from build123d import *

# Parameters (mm, degrees)
F1_DEPTH = 25.4
F2_R     = 5.08
F3_R     = 5.08
F4_R     = 8.3693802945
F5_DEPTH = 99.314


with BuildPart() as f1:
    # F0 (on Front) → F1 (new body, symmetric)
    with BuildSketch(Plane.XZ):
        Polygon((37.378333509, -16.5805853903), (37.378333509, 16.5805853903), (9.2585918344, 16.5805853903), (-10.9242624321, 16.5805853903), (-37.378333509, 16.5805853903), (-37.378333509, -16.5805853903), align=None)
        with BuildLine():
            Line((-10.9242624321, 16.5805853903), (9.2585918344, 16.5805853903))
            ThreePointArc((9.2585918344, 16.5805853903), (16.1053006485, 34.9702005239), (33.311298198, 44.4046594203))
            Line((33.311298198, 44.4046594203), (33.311298198, 64.7116564196))
            ThreePointArc((33.311298198, 64.7116564196), (1.814383096, 49.2661510986), (-10.9242624321, 16.5805853903))
        make_face()
        with BuildLine():
            Line((33.311298198, 72.2287222743), (33.311298198, 64.7116564196))
            ThreePointArc((33.311298198, 64.7116564196), (57.7910346378, 60.35800431), (76.8620222807, 44.4046594203))
            Line((76.8620222807, 44.4046594203), (76.8620222807, 72.2287222743))
            Line((76.8620222807, 72.2287222743), (33.311298198, 72.2287222743))
        make_face()
        with BuildLine():
            Line((33.311298198, 64.7116564196), (33.311298198, 44.4046594203))
            Line((33.311298198, 44.4046594203), (76.8620222807, 44.4046594203))
            ThreePointArc((76.8620222807, 44.4046594203), (57.7910346378, 60.35800431), (33.311298198, 64.7116564196))
        make_face()
    extrude(amount=F1_DEPTH, both=True)

    # F2
    f2_edges = [f1.edges().sort_by_distance(p)[0] for p in [
        (-37.378334, -25.4, 0),
        (37.378334, -25.4, 0),
        (37.378334, 25.4, 0),
        (-37.378334, 25.4, 0),
    ]]
    fillet(f2_edges, radius=F2_R)

    # F3
    f3_edges = [f1.edges().sort_by_distance(p)[0] for p in [
        (9.258592, 0, 16.580585),
        (-10.924262, 0, 16.580585),
        (33.311298, 0, 72.228722),
        (76.862022, 0, 72.228722),
        (76.862022, 0, 44.404659),
    ]]
    fillet(f3_edges, radius=F3_R)

    # F4 (on face) → F5 (cut)
    with BuildSketch(Plane(origin=(0, 0, -16.5805853903), x_dir=(1, 0, 0), z_dir=(0, 0, -1))):
        Circle(F4_R)
    extrude(amount=-F5_DEPTH, mode=Mode.SUBTRACT)


solid = f1.part
Check sheet for the modelled part. Datum: model origin and axes. Units: mm. A direction names the side the tool comes from. Give positions to 0.01 mm unless a question says otherwise; leave off trailing zeros. Order: outer loops, then holes, each group sorted by start corner. A loop starts at its lowest first (then second) coordinate and runs counter-clockwise, first axis right, second up. Notation, with made-up numbers: M 76,40.25 L 82,40.25 A25 ccw 82,58.25 Z; hole C 5,-32 d4. An arc over 180 degrees is marked long. Answer as CSV lines item,"result". Start each with the question number.
Item 1: Thickness scan on line 1 (Y direction, x = 0, z = 25); line 2 (X direction, y = 0, z = 12); line 3 (X direction, y = 0, z = 22.5). Record the ranges inside material, lowest first. Write a range as [from, to].
Item 2: Cross-section at D-D on y = 17.5. Enter the section's corners in (x, z), plus the area to 3 significant figures.
Item 3: Mould release check, pull along Y, two halves, no side actions. Record for faces 5 (the face through (9, -25.4, 28)), 6 (the face through (33.311, 0, 66)), 7 (the face through (7.983, -2.514, 18.808)), 8 (the face through (-35.9, 23.9, -0.2)): +Y half, -Y half, draft (parallel to the pull), parting line (faces both ways), or undercut.
Item 4: Tool access check on faces 1 (the face through (-37.378, 0, 0)), 2 (the face through (26, 0, 16.581)), 3 (the face through (35.9, 23.9, 0.2)), 4 (the face through (37.378, 0, 0)). Record the directions out of +Z, -Z, +X, -X, +Y, -Y that give a thin tool (end or side, any length) a straight path to the whole face; none if there is none.
Item 5: Cross-section at C-C on x = 0. Enter the section's corners in (y, z).
Item 6: Cross-section at A-A on z = 12. Enter the section's corners in (x, y), plus the area to 3 significant figures.
Item 7: Gauge pin test, flat ends, axial feed: P1, Ø12, axis at x = 31.5, y = 17.5, coming from the +Z side; P2, Ø17.5, axis at x = -22.5, y = -5, coming from the +Z side; P3, Ø1.5, axis at x = 7, y = -20, coming from the +Z side. Record the tip position at first contact, or that the pin passes through.
Item 8: Cross-section at B-B on y = 0. Enter the section's corners in (x, z), plus the area to 3 significant figures.
Established:
1,line 1,"y = [-25.4, -8.37], [8.37, 25.4]"
1,line 2,"x = [-37.38, -8.37], [8.37, 37.38]"
1,line 3,"x = [-10.56, -8.37], [8.37, 9.9]"
2,outline,"M -37.38,-16.58 L 37.38,-16.58 L 37.38,16.58 L 14.91,16.58 A5.08 cw 9.95,22.78 A28.12 cw 33.31,44.4 L 71.78,44.4 A5.08 ccw 76.86,49.48 L 76.86,67.15 A5.08 ccw 71.78,72.23 L 38.39,72.23 A5.08 ccw 33.31,67.15 L 33.31,64.71 A48.3 ccw -10.71,21.18 A5.08 cw -15.76,16.58 L -37.38,16.58 Z"
2,area,"4,820 mm^2"
3,face 5,"-Y half"
3,face 6,"draft"
3,face 7,"undercut"
3,face 8,"+Y half"
4,face 1,"+Z, -Z, -X, +Y, -Y"
4,face 2,"+X, +Y, -Y"
4,face 3,"-Z, +X, +Y"
4,face 4,"-Z, +X, +Y, -Y"
5,outline,"M -25.4,-16.58 L -8.37,-16.58 L -8.37,47.17 L -25.4,47.17 Z; M 8.37,-16.58 L 25.4,-16.58 L 25.4,47.17 L 8.37,47.17 Z"
6,outline,"M -37.38,-20.32 A5.08 ccw -32.3,-25.4 L 32.3,-25.4 A5.08 ccw 37.38,-20.32 L 37.38,20.32 A5.08 ccw 32.3,25.4 L -32.3,25.4 A5.08 ccw -37.38,20.32 Z; hole C 0,0 d16.74"
6,area,"3,560 mm^2"
7,P1,"stops at z = 72.15"
7,P2,"stops at z = 17"
7,P3,"stops at z = 54.73"
8,outline,"M -37.38,-16.58 L -8.37,-16.58 L -8.37,32.08 A48.3 ccw -10.71,21.18 A5.08 cw -15.76,16.58 L -37.38,16.58 Z; M 8.37,-16.58 L 37.38,-16.58 L 37.38,16.58 L 14.91,16.58 A5.08 cw 9.95,22.78 A28.12 cw 33.31,44.4 L 71.78,44.4 A5.08 ccw 76.86,49.48 L 76.86,67.15 A5.08 ccw 71.78,72.23 L 38.39,72.23 A5.08 ccw 33.31,67.15 L 33.31,64.71 A48.3 ccw 8.37,55.2 Z"
8,area,"3,770 mm^2"
